Build history of the part. All positions in model axes, mm. A direction names the side the tool comes from. Give positions to 0.01 mm unless a question says otherwise; leave off trailing zeros. Loops run counter-clockwise (first coordinate to the right, second up) from the corner with the lowest first, then second, coordinate; pieces in that order, holes last. Notation, with made-up numbers: M 42,-16 L 47,-16 A15 ccw 47,9 Z; hole C -10.75,15 d6. An arc over 180 degrees is marked long. Answer as a JSON object with one key per item and string values. Group by question number.
1. Slice it at B-B (z = 14). List the corners of the cut face in (x, y), then the cut area to 3 significant figures.
2. Drill centre lines: line 1 along Y through (x, z) = (-0.5, 2.75); line 2 along Z through (x, y) = (0.65, 0.15). Where is each one in solid material? Low to high. Write a range as [from, to].
3. 3-axis set-ups, long thin cutter, end or side, ignore diameter. For faces 4 (the face through (-0.44, 0.02, 10.69)), 5 (the face through (-0.2, 1, 18)), 6 (the face through (0.2, -1, 2)), 7 (the face through (0.2, 1, 18)): which of +Z, -Z, +X, -X, +Y, -Y reach the whole face in a straight line?
4. Slice it at A-A (x = -1.4). List the corners of the cut face in (y, z), then the cut area to 3 significant figures.
5. Drop flat-ended pins along their axis: pin 1 Ø1 at (y, z) = (0, 9) entering from +X; pin 2 Ø1.1 at (y, z) = (1, 2) entering from -X; pin 3 Ø0.7 at (x, z) = (1, 3) entering from +Y. Give the stop position or say it passes through.
6. Mould opens along Z. For faces 1 (the face through (-1.1, 0, 3.9)), 2 (the face through (-0.2, 1, 2)), 3 (the face through (0, 0, 0)) say: released by +Z, released by -Z, zero draft, split by the parting line, or undercut.
7. Slice it at C-C (x = 0). List the corners of the cut face in (y, z).
from build123d import *

# Parameters (mm, degrees)
F3_DEPTH = 0.2
F4_COUNT = 4


# Not quite as in the source:
# - a feature names something its author has since deleted; it is built from what else it names


with BuildPart() as f1:
    # F0 (on Front) → F1 (revolve)
    with BuildSketch(Plane.XZ):
        with BuildLine():
            Line((0, 21.5277777778), (0, 0))
            Line((0, 0), (0.4409722222, 0))
            Line((0.4409722222, 0), (0.4409722222, 21.0868055556))
            ThreePointArc((0.4409722222, 21.0868055556), (0.3118144486, 21.3986200042), (0, 21.5277777778))
        make_face()
    revolve(axis=Axis((0, 0, 10.7638888889), (0, 0, 1)))

    # F2 (on Front) → F3 (join, symmetric)
    with BuildSketch(Plane.XZ):
        Polygon((0, 18.4355709877), (0, 17.8472222222), (2.0138888889, 17.8472222222), (2.0138888889, 18.6111111111), (1.1805555556, 19.0972222222), (0.7534722222, 20.1388888889), (0.7534722222, 18.8541666667), align=None)
        Polygon((0, 4.8655856243), (0, 0.3819444444), (1.7881944444, 0.3819444444), (1.7881944444, 3.2986111111), align=None)
    extrude(amount=F3_DEPTH, both=True)

    # F4: F1 ×4 about axis
    f4_axis = Axis((0, 0, 0), (0, 0, 1))


with BuildPart() as f1_1:
    add(f1.part)
    for i in range(1, F4_COUNT):
        add(f1.part.rotate(f4_axis, i * 360 / F4_COUNT))


solid = f1_1.part
Established:
{
 "1": {"outline": "C 0,0 d0.88", "area": "0.611 mm^2"},
 "2": {"line 1": "y = [-0.2, 0.2]", "line 2": "z = [0.38, 4.3], [17.85, 18.8]"},
 "3": {"face 4": "none", "face 5": "+Z, -Z, -X, +Y", "face 6": "+Z, -Z, +X, -Y", "face 7": "+Z, -Z, +X, +Y"},
 "4": {"outline": "M -0.2,0.38 L 0.2,0.38 L 0.2,3.64 L -0.2,3.64 Z; M -0.2,17.85 L 0.2,17.85 L 0.2,18.97 L -0.2,18.97 Z", "area": "1.75 mm^2"},
 "5": {"pin 1": "stops at x = 0.44", "pin 2": "stops at x = -0.2", "pin 3": "stops at y = 0.2"},
 "6": {"face 1": "undercut", "face 2": "zero draft", "face 3": "released by -Z"},
 "7": {"outline": "M -2.01,17.85 L -0.44,17.85 L -0.44,4.48 L -1.79,3.3 L -1.79,0.38 L -0.44,0.38 L -0.44,0 L 0.44,0 L 0.44,0.38 L 1.79,0.38 L 1.79,3.3 L 0.44,4.48 L 0.44,17.85 L 2.01,17.85 L 2.01,18.61 L 1.18,19.1 L 0.75,20.14 L 0.75,18.85 L 0.44,18.68 L 0.44,21.09 A0.44 ccw -0.44,21.09 L -0.44,18.68 L -0.75,18.85 L -0.75,20.14 L -1.18,19.1 L -2.01,18.61 Z"}
}
